from build123d import *

# Parameters (mm, degrees)
SKETCH1_R           = 7.5
BOSS_EXTRUDE1_DEPTH = 10


with BuildPart() as part:
    # Sketch1 → Boss-Extrude1 (new body)
    with BuildSketch(Plane(origin=(0, 0, 0), x_dir=(0, 0, -1), z_dir=(1, 0, 0))):
        with BuildLine():
            Line((-15, -20), (15, -20))
            Line((15, -20), (15, 0))
            ThreePointArc((15, 0), (0, 15), (-15, 0))
            Line((-15, 0), (-15, -20))
        make_face()
        Circle(SKETCH1_R, mode=Mode.SUBTRACT)
    extrude(amount=BOSS_EXTRUDE1_DEPTH)


solid = part.part
Here's how the part is built. I have some questions about the finished solid (model axes, mm). Coordinates: 2 decimals unless noted, no trailing zeros. Write each loop counter-clockwise with the first axis right and the second up, starting at its lowest first coordinate (ties: lowest second). Pieces come first, ordered by that corner, then holes.
1) If we section it at B-B (y = -5): List the corners of the cut face in (x, z) for me.
Filled in:
outline: (0, -15) - (10, -15) - (10, -5.59) - (0, -5.59) - close; (0, 5.59) - (10, 5.59) - (10, 15) - (0, 15) - close
2) If we section it at C-C (x = 1.25): List the corners of the cut face in (y, z) for me, plus the area to 3 significant figures.
Filled in:
outline: (-20, -15) - (0, -15) arc R15 ccw to (0, 15) - (-20, 15) - close; hole circle Ø15 at (0, 0)
area: 777 mm2
3) If we section it at A-A (z = 0): List the corners of the cut face in (x, y) for me.
Filled in:
outline: (0, -20) - (10, -20) - (10, -7.5) - (0, -7.5) - close; (0, 7.5) - (10, 7.5) - (10, 15) - (0, 15) - close
4) If we section it at D-D (y = 12): List the corners of the cut face in (x, z) for me, plus the area to 3 significant figures.
Filled in:
outline: (0, -9) - (10, -9) - (10, 9) - (0, 9) - close
area: 180 mm2
5) I'm going to push a flat-ended pin straight in: pin 1 (3 mm diameter, centred on x = 9, z = -0.5, fed in from +Y). Where does the tip first touch, or does it pass through?
Filled in:
pin 1: stops at y = 15
6) Thinking about a two-plate mould opening in Z: for faces 1 (the face through (5, -10, -15)), 2 (the face through (4.93, 0.33, 7.493)), 3 (the face through (5, -20, 0)), 4 (the face through (5, -10, 15)), which applies, +Z half, -Z half, draft (parallel to the pull), parting line (faces both ways), or undercut?
Filled in:
face 1: -Z half
face 2: undercut
face 3: draft
face 4: +Z half
7) If I drill on line 1 (Y direction, x = 5.5, z = 0); line 2 (Z direction, x = 8.75, y = 6); line 3 (Y direction, x = 7.5, z = -5), over which ranges is the centre line in solid material (lowest first)?
Filled in:
line 1: y = -20 to -7.5, 7.5 to 15
line 2: z = -13.75 to -4.5, 4.5 to 13.75
line 3: y = -20 to -5.59, 5.59 to 14.14
